```python
from build123d import *

# Parameters (mm, degrees)
BOSS_EXTRUDE1_DEPTH = 4
CHAMFER1_SIZE       = 6
SKETCH2_R           = 0.357314597
CUT_EXTRUDE1_DEPTH  = 1


with BuildPart() as part:
    # Sketch1 → Boss-Extrude1 (new body)
    with BuildSketch(Plane.XY):
        with BuildLine():
            Line((-193.5, 5), (-193.5, 13.029022597))
            Line((-193.5, 13.029022597), (-190.028351822, 16.768866664))
            Line((-190.028351822, 16.768866664), (-192.886698165, 19.422232071))
            Line((-192.886698165, 19.422232071), (-193.593804946, 19.422232071))
            Line((-193.593804946, 19.422232071), (-194.318589397, 20.147016522))
            Line((-194.318589397, 20.147016522), (-190.783055491, 23.682550428))
            Line((-190.783055491, 23.682550428), (-189.351164259, 22.250659196))
            Line((-189.351164259, 22.250659196), (-188.997610869, 22.604212587))
            Line((-188.997610869, 22.604212587), (-189.527940955, 23.134542672))
            Line((-189.527940955, 23.134542672), (-187.760174002, 24.902309625))
            Line((-187.760174002, 24.902309625), (-188.661735148, 25.803870771))
            Line((-188.661735148, 25.803870771), (-187.954628366, 26.510977553))
            Line((-187.954628366, 26.510977553), (-190.040593371, 28.596942557))
            Line((-190.040593371, 28.596942557), (-190.747700152, 27.889835776))
            Line((-190.747700152, 27.889835776), (-191.649261298, 28.791396922))
            Line((-191.649261298, 28.791396922), (-193.417028251, 27.023629969))
            Line((-193.417028251, 27.023629969), (-193.947358337, 27.553960055))
            Line((-193.947358337, 27.553960055), (-194.300911728, 27.200406664))
            Line((-194.300911728, 27.200406664), (-192.869020496, 25.768515432))
            Line((-192.869020496, 25.768515432), (-196.404532161, 22.233003767))
            Line((-196.404532161, 22.233003767), (-197.129316611, 22.957788218))
            Line((-197.129316611, 22.957788218), (-197.129316611, 23.664894999))
            Line((-197.129316611, 23.664894999), (-198.543530174, 25.079108562))
            ThreePointArc((-198.543530174, 25.079108562), (-199.69683639, 30.30316361), (-204.920891438, 31.456469826))
            Line((-204.920891438, 31.456469826), (-206.335105001, 32.870683389))
            Line((-206.335105001, 32.870683389), (-207.042211782, 32.870683389))
            Line((-207.042211782, 32.870683389), (-207.766996233, 33.595467839))
            Line((-207.766996233, 33.595467839), (-204.231484568, 37.130979504))
            Line((-204.231484568, 37.130979504), (-202.799593336, 35.699088272))
            Line((-202.799593336, 35.699088272), (-202.446039945, 36.052641663))
            Line((-202.446039945, 36.052641663), (-202.976370031, 36.582971749))
            Line((-202.976370031, 36.582971749), (-201.208603078, 38.350738702))
            Line((-201.208603078, 38.350738702), (-202.110164224, 39.252299848))
            Line((-202.110164224, 39.252299848), (-201.403057443, 39.959406629))
            Line((-201.403057443, 39.959406629), (-203.489022447, 42.045371634))
            Line((-203.489022447, 42.045371634), (-204.196129229, 41.338264852))
            Line((-204.196129229, 41.338264852), (-205.097690375, 42.239825998))
            Line((-205.097690375, 42.239825998), (-206.865457328, 40.472059045))
            Line((-206.865457328, 40.472059045), (-207.395787413, 41.002389131))
            Line((-207.395787413, 41.002389131), (-207.749340804, 40.648835741))
            Line((-207.749340804, 40.648835741), (-206.317449572, 39.216944509))
            Line((-206.317449572, 39.216944509), (-209.852983478, 35.681410603))
            Line((-209.852983478, 35.681410603), (-210.577767929, 36.406195054))
            Line((-210.577767929, 36.406195054), (-210.577767929, 37.113301835))
            Line((-210.577767929, 37.113301835), (-212.026855734, 38.56238964))
            Line((-212.026855734, 38.56238964), (-212.026855734, 41.337590552))
            Line((-212.026855734, 41.337590552), (-209.789156947, 43.57528934))
            ThreePointArc((-209.789156947, 43.57528934), (-203.686966217, 46.169596994), (-197.492575262, 43.803865688))
            Line((-197.492575262, 43.803865688), (-160, 9))
            Line((-160, 9), (-160, 5))
            Line((-160, 5), (-10, 5))
            Line((-10, 5), (-10, 9))
            Line((-10, 9), (0, 9))
            Line((0, 9), (0, 5))
            Line((0, 5), (20, 5))
            Line((20, 5), (20, 0))
            Line((20, 0), (0, 0))
            Line((0, 0), (0, -10))
            Line((0, -10), (-243.5, -10))
            Line((-243.5, -10), (-243.5, -1))
            Line((-243.5, -1), (-249.5, 5))
            Line((-249.5, 5), (-249.5, 9))
            Line((-249.5, 9), (-239.5, 9))
            Line((-239.5, 9), (-239.5, 5))
            Line((-239.5, 5), (-193.5, 5))
        make_face()
    extrude(amount=BOSS_EXTRUDE1_DEPTH)

    # Chamfer1
    chamfer1_edges = [part.edges().sort_by_distance(p)[0] for p in [
        (0, -10, 2),
    ]]
    chamfer(chamfer1_edges, length=CHAMFER1_SIZE)

    # Sketch2 → Cut-Extrude1 (cut)
    with BuildSketch(Plane(origin=(-80.721825407, -80.721825407, 0), x_dir=(0, 0, 1), z_dir=(-0.7071067811865454, -0.7071067811865497, 0))):
        with Locations(Location((2, 172.10347727, 0), (0, 0, 270))):
            Circle(SKETCH2_R)
        with Locations(Location((2, 153.121208308, 0), (0, 0, 270))):
            Circle(SKETCH2_R)
    extrude(amount=-CUT_EXTRUDE1_DEPTH, mode=Mode.SUBTRACT)


solid = part.part
```
Here's how the part is built. I have some questions about the finished solid (model axes, mm). Give positions to 0.01 mm unless a question says otherwise; leave off trailing zeros. Write each loop counter-clockwise with the first axis right and the second up, starting at its lowest first coordinate (ties: lowest second). Pieces come first, ordered by that corner, then holes. Notation, with made-up numbers: (78, 24) -> (123, 24) arc R16 ccw to (123, 31) -> close; hole circle Ø5 at (-1, 79). An arc over 180 degrees is marked (long way). Use one line per item in the form item = value.
1) If I drill on L1, parallel to X at y = 7, z = 0.25; L2, parallel to Y at x = -204.5, z = 0.4; L3, parallel to Y at x = -52.5, z = 3.05, over which ranges is the centre line in solid material (lowest first)? Write a range as [from, to].
Verdict:
L1 = [-249.5, -239.5], [-193.5, -160], [-10, 0]
L2 = [-10, 5], [31.59, 36.86], [41.64, 46.12]
L3 = [-10, 5]
2) Suppose I cut it at A-A (x = -61). Please give me the cut outline in (y, z).
Verdict:
outline = (-10, 0) -> (5, 0) -> (5, 4) -> (-10, 4) -> close
3) Suppose I cut it at B-B (x = -170). Please give me the cut outline in (y, z), and give its area (3 significant figures).
Verdict:
outline = (-10, 0) -> (18.28, 0) -> (18.28, 4) -> (-10, 4) -> close
area = 113 mm2
4) We'd pull the mould along Y, two halves only. Please class faces 1 (the face through (-199.641, 30.247, 1.972)), 2 (the face through (-3, -7, 2)), 3 (the face through (-179.009, 26.646, 1.972)), 4 (the face through (-134, -1, 4)): +Y half, -Y half, draft (parallel to the pull), parting line (faces both ways), or undercut.
Verdict:
face_1 = undercut
face_2 = -Y half
face_3 = +Y half
face_4 = draft
5) I'm going to push flat-ended pins straight in: pin 1 (0.6 mm diameter, centred on y = 23.5, z = 2.5, fed in from -X); pin 2 (1.2 mm diameter, centred on y = 6.5, z = 2.5, fed in from +X); pin 3 (2 mm diameter, centred on y = 19, z = 1.5, fed in from -X). Where does each tip first touch, or does it pass through?
Verdict:
pin_1 = -197.26
pin_2 = 0
pin_3 = -194.17
